Build history of the part. All positions in model axes, mm. A direction names the side the tool comes from. Give positions to 0.01 mm unless a question says otherwise; leave off trailing zeros. Order: outer loops, then holes, each group sorted by start corner. A loop starts at its lowest first (then second) coordinate and runs counter-clockwise, first axis right, second up. Notation, with made-up numbers: (23, 5.5) -> (39, 5.5) arc R37 cw to (39, 44.5) -> close; hole circle Ø1 at (-0.5, -4.5). An arc over 180 degrees is marked (long way). Use a Markdown table: item, result. Add a question column.
```python
from build123d import *

# Parameters (mm, degrees)
SKETCH_2_R          = 5.5
EXTRUDE_1_DEPTH     = 4
SKETCH_3_R          = 4.5
EXTRUDE_2_DEPTH     = 7
SKETCH_4_R          = 3.5
CUT_EXTRUDE_1_DEPTH = 4.5
FILLET_1_R          = 0.4
FILLET_2_R          = 0.2


with BuildPart() as part:
    # 草图2 → 凸台-拉伸1 (new body)
    with BuildSketch(Plane(origin=(0, 0, 0), x_dir=(1, 0, 0), z_dir=(0, 1, 0))):
        Circle(SKETCH_2_R)
    extrude(amount=EXTRUDE_1_DEPTH)

    # 草图3 → 凸台-拉伸2 (add)
    with BuildSketch(Plane(origin=(0, 4, 0), x_dir=(1, 0, 0), z_dir=(0, 1, 0))):
        Circle(SKETCH_3_R)
    extrude(amount=EXTRUDE_2_DEPTH)

    # 草图4 → 切除-拉伸1 (cut)
    with BuildSketch(Plane.XZ):
        Circle(SKETCH_4_R)
    extrude(amount=-CUT_EXTRUDE_1_DEPTH, mode=Mode.SUBTRACT)

    # 圆角1
    fillet_1_edges = [part.edges().sort_by_distance(p)[0] for p in [
        (-3.5, 0, 0),
        (-5.5, 0, 0),
        (-4.5, 11, 0),
    ]]
    fillet(fillet_1_edges, radius=FILLET_1_R)

    # 圆角2
    fillet_2_edges = [part.edges().sort_by_distance(p)[0] for p in [
        (-5.5, 4, 0),
        (-4.5, 4, 0),
    ]]
    fillet(fillet_2_edges, radius=FILLET_2_R)


solid = part.part
```
(1) Band-saw the part on B-B on z = 0. Give the cut face in (x, y).
(2) Tool access for faces 1 (the face through (-1, 0, 4)), 2 (the face through (0, 4, 5)), 3 (the face through (0, 4.5, 0)): list every direction of +Z, -Z, +X, -X, +Y, -Y with a clear straight run to the whole face (end or side of a thin tool).
(3) Wall check: probe 1 along Z at (x, y) = (0, 2.8); probe 2 along Y at (x, z) = (-2.5, 4.25); probe 3 along X at (y, z) = (0.75, -2.25). Give the ranges that are in metal, low to high.
(4) Band-saw the part on A-A on x = 0. Give the cut face in (y, z).
(5) Pin check, flat tips, straight feed: pin 1 Ø3 at (x, y) = (1, 8.5) entering from -Z; pin 2 Ø3 at (y, z) = (9.5, 0) entering from +X; pin 3 Ø2 at (x, y) = (-2.5, 8.5) entering from -Z. Stop position of each tip, or through.
(6) Band-saw the part on D-D on y = 2.5. Give the cut face in (x, z).
(7) Band-saw the part on C-C on y = 7.5. Give the cut face in (x, z).
Response:
| question | item | result |
|---|---|---|
| 1 | outline | (-5.5, 0.4) arc R0.4 ccw to (-5.1, 0) -> (-3.9, 0) arc R0.4 ccw to (-3.5, 0.4) -> (-3.5, 4.5) -> (3.5, 4.5) -> (3.5, 0.4) arc R0.4 ccw to (3.9, 0) -> (5.1, 0) arc R0.4 ccw to (5.5, 0.4) -> (5.5, 3.8) arc R0.2 ccw to (5.3, 4) -> (4.7, 4) arc R0.2 cw to (4.5, 4.2) -> (4.5, 10.6) arc R0.4 ccw to (4.1, 11) -> (-4.1, 11) arc R0.4 ccw to (-4.5, 10.6) -> (-4.5, 4.2) arc R0.2 cw to (-4.7, 4) -> (-5.3, 4) arc R0.2 ccw to (-5.5, 3.8) -> close |
| 2 | face 1 | +Z, -Z, +X, -X, -Y |
| 2 | face 2 | +Y |
| 2 | face 3 | -Y |
| 3 | probe 1 | z = -5.5 to -3.5, 3.5 to 5.5 |
| 3 | probe 2 | y = 0 to 4 |
| 3 | probe 3 | x = -5.02 to -2.68, 2.68 to 5.02 |
| 4 | outline | (0, -5.1) arc R0.4 ccw to (0.4, -5.5) -> (3.8, -5.5) arc R0.2 ccw to (4, -5.3) -> (4, -4.7) arc R0.2 cw to (4.2, -4.5) -> (10.6, -4.5) arc R0.4 ccw to (11, -4.1) -> (11, 4.1) arc R0.4 ccw to (10.6, 4.5) -> (4.2, 4.5) arc R0.2 cw to (4, 4.7) -> (4, 5.3) arc R0.2 ccw to (3.8, 5.5) -> (0.4, 5.5) arc R0.4 ccw to (0, 5.1) -> (0, 3.9) arc R0.4 ccw to (0.4, 3.5) -> (4.5, 3.5) -> (4.5, -3.5) -> (0.4, -3.5) arc R0.4 ccw to (0, -3.9) -> close |
| 5 | pin 1 | stops at z = -4.5 |
| 5 | pin 2 | stops at x = 4.5 |
| 5 | pin 3 | stops at z = -4.24 |
| 6 | outline | circle Ø11 at (0, 0); hole circle Ø7 at (0, 0) |
| 7 | outline | circle Ø9 at (0, 0) |
